Input: part model. Units: mm. Frame: model coordinates. Face numbers are marked on the shaded views. A direction names the side the tool comes from. Round coordinates to 2 decimals unless told otherwise and drop trailing zeros. Loops run counter-clockwise (first coordinate to the right, second up) from the corner with the lowest first, then second, coordinate; pieces in that order, holes last. Notation, with made-up numbers: M 85,72.5 L 126,72.5 A17 cw 126,84.5 Z; hole C 15.5,-15.5 d3. An arc over 180 degrees is marked long. Return JSON: item names as keys, results as strings. Group by question number.
1) Material intervals for line 1 (X direction, y = -4.5, z = -12); line 2 (Z direction, x = 5.5, y = -3.5); line 3 (X direction, y = 6.25, z = -23.5), sorted ascending. Write a range as from..to.
2) Section D-D (x = -7). Output: boundary loops of the cut face in (y, z), plus the area to 3 significant figures.
3) Contact query for flat-ended pins moving along their axis: P1, Ø12, axis at y = -6.5, z = -12.5, coming from the -X side; P2, Ø1, axis at x = -4, y = -8, coming from the +Z side; P3, Ø6, axis at y = 0, z = -20, coming from the -X side; P4, Ø5, axis at x = 4.5, y = -4, coming from the -Z side. Output: stop coordinate, or through.
4) Section A-A (x = -19). Output: boundary loops of the cut face in (y, z).
5) Section B-B (z = -9). Output: boundary loops of the cut face in (x, y), plus the area to 3 significant figures.
6) Mould query, pull axis X, two halves, no side actions, for the marked faces 1, 2, 3 and 4. Classes: +X half, -X half, draft (parallel to the pull), parting line (faces both ways), or undercut.
7) Access query for the marked faces 5, 6, 7 and 8. Directions: +Z, -Z, +X, -X, +Y, -Y. A direction counts if a zero-diameter tool reaches every point of the face in a straight line with its end or side. Return the directions, or none.
8) Section C-C (y = 7). Output: boundary loops of the cut face in (x, z), plus the area to 3 significant figures.
from build123d import *

# Parameters (mm, degrees)
F0_W          = 3
F0_H          = 3
F0_W_2        = 4.5
F0_W_3        = 25
F1_DEPTH      = 10
F1_DEPTH_BACK = 10
F4_DEPTH      = 10
F4_DEPTH_BACK = 10
F5_R          = 6


with BuildPart() as f1:
    # F0 (on Front) → F1 (new body, two sides)
    with BuildSketch(Plane.XZ) as f1_sk:
        with Locations((1.5, 1.5)):
            Rectangle(F0_W, F0_H)
        Polygon((3, 0), (0, 0), (0, -27), (0, -30), (3, -30), align=None)
        with Locations((5.25, 1.5)):
            Rectangle(F0_W_2, F0_H)
        with Locations((-12.5, -28.5)):
            Rectangle(F0_W_3, F0_H)
        Polygon((7.5, 3), (7.5, 0), (7.5, -30), (10.5, -30), (10.5, 3), align=None)
    extrude(amount=F1_DEPTH)
    extrude(f1_sk.sketch, amount=-F1_DEPTH_BACK)

    # F3 (on offset) → F4 (cut, two sides)
    with BuildSketch(Plane.XY.offset(-20)) as f4_sk:
        with BuildLine():
            ThreePointArc((-15, -5), (-11.464466, -3.535534), (-10, 0))
            Line((-10, 0), (-25, 0))
            Line((-25, 0), (-25, -5))
            Line((-25, -5), (-15, -5))
        make_face()
        with BuildLine():
            Line((-25, 0), (-10, 0))
            ThreePointArc((-10, 0), (-11.464466, 3.535534), (-15, 5))
            Line((-15, 5), (-25, 5))
            Line((-25, 5), (-25, 0))
        make_face()
    extrude(amount=F4_DEPTH, mode=Mode.SUBTRACT)
    extrude(f4_sk.sketch, amount=-F4_DEPTH_BACK, mode=Mode.SUBTRACT)

    # F5
    f5_edges = [f1.edges().sort_by_distance(p)[0] for p in [
        (0, 0, -27),
    ]]
    fillet(f5_edges, radius=F5_R)


solid = f1.part
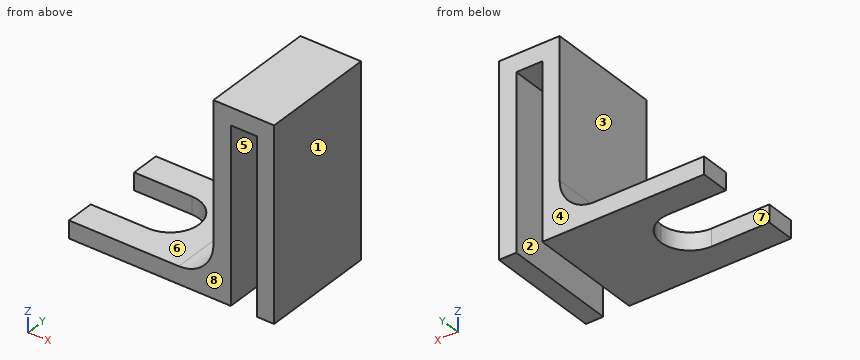
Returned:
{
 "1": {"line 1": "x = 0..3, 7.5..10.5", "line 2": "z = 0..3", "line 3": "x = -0.55..3, 7.5..10.5"},
 "2": {"outline": "M -10,-30 L 10,-30 L 10,-27 L -10,-27 Z", "area": "60.0 mm^2"},
 "3": {"P1": "stops at x = 0", "P2": "stops at z = -26.45", "P3": "stops at x = -0.34", "P4": "stops at z = -30"},
 "4": {"outline": "M -10,-30 L -5,-30 L -5,-27 L -10,-27 Z; M 5,-30 L 10,-30 L 10,-27 L 5,-27 Z"},
 "5": {"outline": "M 0,-10 L 3,-10 L 3,10 L 0,10 Z; M 7.5,-10 L 10.5,-10 L 10.5,10 L 7.5,10 Z", "area": "120 mm^2"},
 "6": {"face 1": "+X half", "face 2": "undercut", "face 3": "-X half", "face 4": "draft"},
 "7": {"face 5": "-Z, +Y, -Y", "face 6": "+Z, -X, +Y, -Y", "face 7": "+Z, -Z, -X", "face 8": "+Z, -Z, +X, -X, -Y"},
 "8": {"outline": "M -25,-30 L 3,-30 L 3,0 L 7.5,0 L 7.5,-30 L 10.5,-30 L 10.5,3 L 0,3 L 0,-21 A6 cw -6,-27 L -25,-27 Z", "area": "294 mm^2"}
}
